from build123d import *

# Parameters (mm, degrees)
F0_W     = 200
F0_H     = 100
F1_DEPTH = 10
F2_R     = 20
F3_DEPTH = 10.001
F4_R     = 4.99999


# Not quite as in the source:
# - a fillet or chamfer is up to 0.001 mm smaller than in the source, because OpenCascade refuses the exact size


with BuildPart() as f1:
    # F0 (on Front) → F1 (new body)
    with BuildSketch(Plane.XZ):
        Rectangle(F0_W, F0_H)
    extrude(amount=F1_DEPTH)

    # F2 (on face) → F3 (cut, through all)
    with BuildSketch(Plane.XZ.offset(10)):
        with Locations((0, -1.9458576571)):
            Circle(F2_R)
    extrude(amount=-F3_DEPTH, mode=Mode.SUBTRACT)

    # F4 (radius 5 in the source; OpenCascade refuses exactly that, so slightly less here)
    f4_edges = [f1.edges().sort_by_distance(p)[0] for p in [
        (0, -10, 50),
        (0, 0, 50),
        (100, 0, 0),
        (100, -10, 0),
        (0, -10, -50),
        (-100, -10, 0),
    ]]
    fillet(f4_edges, radius=F4_R)


solid = f1.part
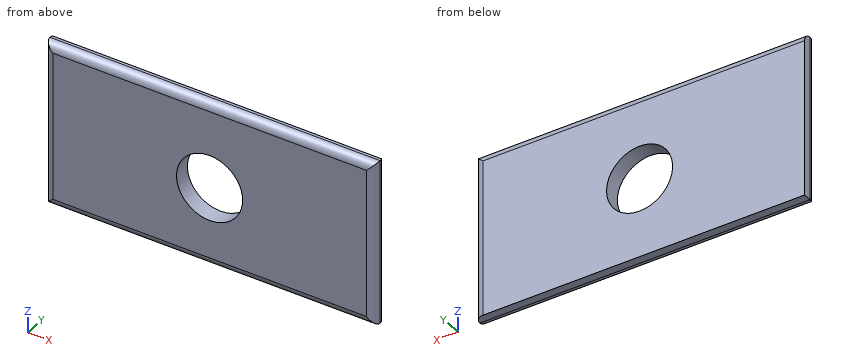
Source: CAD feature listing. Evaluate the final solid. Frame: model axes, mm. Round coordinates to 2 decimals unless told otherwise and drop trailing zeros. Loops run counter-clockwise (first coordinate to the right, second up) from the corner with the lowest first, then second, coordinate; pieces in that order, holes last. Notation, with made-up numbers: M 57.25,23 L 63.25,23 A20 ccw 63.25,40 Z; hole C 15,46 d3. An arc over 180 degrees is marked long. Return JSON: item names as keys, results as strings. Group by question number.
1. Material intervals for line 1 along X through (y, z) = (-1, 0); line 2 along Z through (x, y) = (0, -3.5); line 3 along Z through (x, y) = (6, -1.5), sorted ascending. Write a range as from..to.
2. Section query D-D on y = -8.5. Output: boundary loops of the cut face in (x, z).
3. Pin query (flat end, axial travel): pin 1 (1 mm diameter, centred on x = -7.5, y = -2, fed in from +Z); pin 2 (4 mm diameter, centred on y = -3.5, z = -1.5, fed in from +X); pin 3 (5 mm diameter, centred on y = -8, z = -16, fed in from -X). Return the tip coordinate at first contact, or that it passes through.
Checks:
{
 "1": {"line 1": "x = -100..-19.91, 19.91..98", "line 2": "z = -50..-21.95, 18.05..49.77", "line 3": "z = -50..-21.02, 17.13..48.57"},
 "2": {"outline": "M -98.57,-48.57 L 98.57,-48.57 L 98.57,48.57 L -98.57,48.57 Z; hole C 0,-1.95 d40"},
 "3": {"pin 1": "stops at z = 49.33", "pin 2": "stops at x = 100", "pin 3": "stops at x = -99.97"}
}
